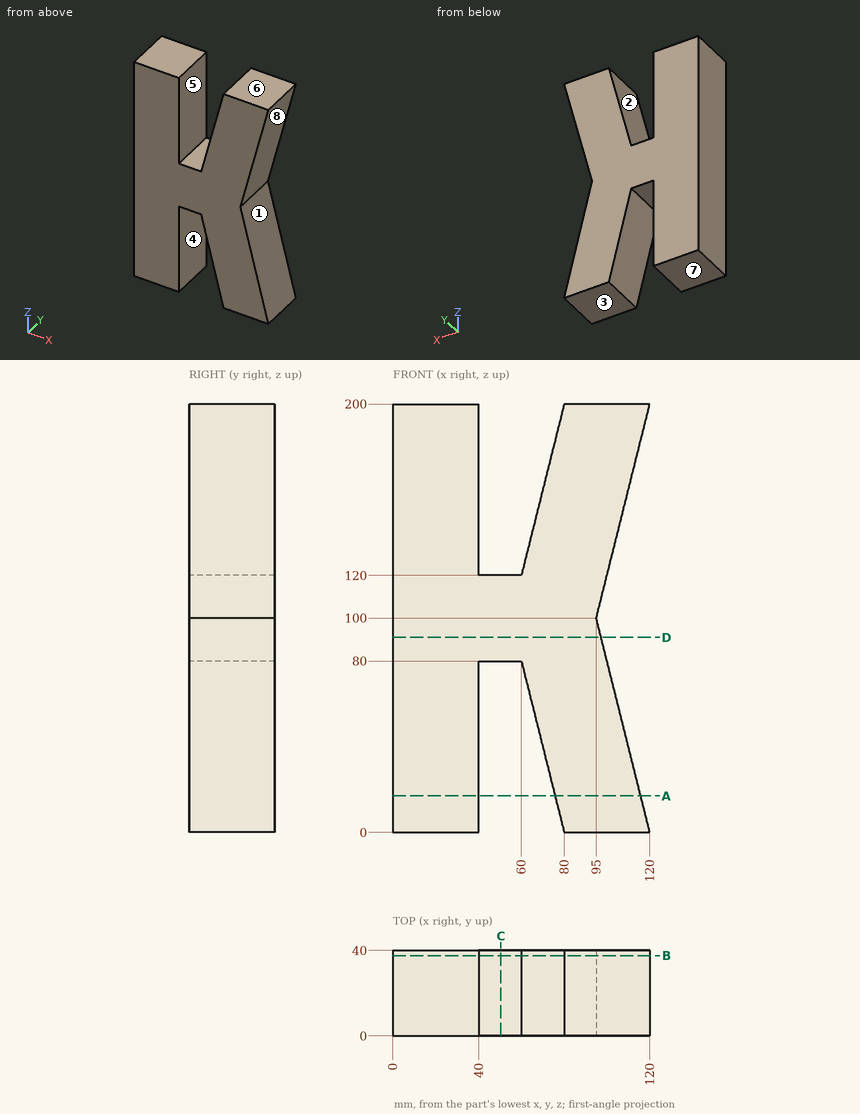
Source: three-view drawing plus pictorial views. Frame: mm from the lowest corner of the part. A direction names the side the tool comes from. Coordinates: 2 decimals unless noted, no trailing zeros. Order: outer loops, then holes, each group sorted by start corner. A loop starts at its lowest first (then second) coordinate and runs counter-clockwise, first axis right, second up.
1) First-contact query: P1, Ø5, axis at y = 21.5, z = 98.5, coming from the +X side; P2, Ø20, axis at y = 27.5, z = 167, coming from the +X side; P3, Ø20, axis at y = 26.5, z = 37.5, coming from the +X side (3 decimals). Flat tips, straight axial feed; report the tip coordinate or a pass-through.
Result sheet:
P1: stops at x = 96
P2: stops at x = 114.25
P3: stops at x = 113.125
2) Ray query, probe 1 along Z at (x, y) = (41.5, 18); probe 2 along X at (y, z) = (5, 24); probe 3 along X at (y, z) = (5.5, 136). Return the intervals inside material, ascending.
Result sheet:
probe 1: z = 80 to 120
probe 2: x = 0 to 40, 74 to 114
probe 3: x = 0 to 40, 64 to 104
3) Set-up query: the marked faces 4, 5, 6, 7 and 8. Return all of +Z, -Z, +X, -X, +Y, -Y with unobstructed straight access to the full face (end or side cutting, diameter ignored); none if empty.
Result sheet:
face 4: -Z, +Y, -Y
face 5: +Z, +Y, -Y
face 6: +Z, +X, -X, +Y, -Y
face 7: -Z, +X, -X, +Y, -Y
face 8: +X, +Y, -Y
4) Draft query along X for the marked faces 1, 2 and 3. Return one class per face: released by +X, released by -X, zero draft, split by the parting line, or undercut.
Result sheet:
face 1: released by +X
face 2: undercut
face 3: zero draft
5) Section D-D (z = 91). Return loops of the section in (x, y).
Result sheet:
outline: (0, 0) - (97.25, 0) - (97.25, 40) - (0, 40) - close
6) Section C-C (x = 50.5). Return loops of the section in (y, z).
Result sheet:
outline: (0, 80) - (40, 80) - (40, 120) - (0, 120) - close
7) Section B-B (y = 37.5). Return loops of the section in (x, z).
Result sheet:
outline: (0, 0) - (40, 0) - (40, 80) - (60, 80) - (80, 0) - (120, 0) - (95, 100) - (120, 200) - (80, 200) - (60, 120) - (40, 120) - (40, 200) - (0, 200) - close
8) Section A-A (z = 17). Return loops of the section in (x, y), then the cut area to 3 significant figures.
Result sheet:
outline: (0, 0) - (40, 0) - (40, 40) - (0, 40) - close; (75.75, 0) - (115.75, 0) - (115.75, 40) - (75.75, 40) - close
area: 3,200 mm2
